Verification items for the finished model (mm, model axes). A direction names the side the tool comes from. Round coordinates to 2 decimals unless told otherwise and drop trailing zeros. Order: outer loops, then holes, each group sorted by start corner. A loop starts at its lowest first (then second) coordinate and runs counter-clockwise, first axis right, second up. Notation, with made-up numbers: M 85.25,-1.5 L 98.25,-1.5 A29 cw 98.25,27.5 Z; hole C 9,48 d2. An arc over 180 degrees is marked long. Use one line per item in the form item = value. Start each with the question number.
Item 1: Thickness scan on probe 1 along Z at (x, y) = (0, 506); probe 2 along Z at (x, y) = (68, 118.5); probe 3 along Y at (x, z) = (-36.5, -3.5). Record the ranges inside material, lowest first. Write a range as [from, to].
Item 2: Release check for a two-part mould opening along X. For faces 3 (the flat face through (-34, 0, -95)), 4 (the cylindrical face through (-89.42, 470.82, 37.07)), 5 (the cylindrical face through (138.304, -3.944, -43.554)), 6 (the flat face through (-1, 0, 1)) record: +X half, -X half, draft (parallel to the pull), parting line (faces both ways), or undercut.
Item 3: Cross-section at C-C on y = 176.5. Enter the section's corners in (x, z).
Item 4: Tool access check on faces 1 (the flat face through (52, 955, 82)), 2 (the cylindrical face through (-95.38, 470.82, -30.04)). Record the directions out of +Z, -Z, +X, -X, +Y, -Y that give a thin tool (end or side, any length) a straight path to the whole face; none if there is none.
Item 5: Cross-section at B-B on x = 0. Enter the section's corners in (y, z).
Item 6: Cross-section at A-A on z = 0. Enter the section's corners in (x, y), then the cut area to 3 significant figures.
Item 7: Go/stop test with flat-tipped pins: pin 1 Ø5 at (x, y) = (89.5, 847) entering from +Z; pin 2 Ø10 at (x, y) = (-10, 223.5) entering from +Z; pin 3 Ø3 at (y, z) = (638, 80.5) entering from +X. Record where each tip stops, or that it passes through.
Item 8: Cross-section at D-D on x = 110.5. Enter the section's corners in (y, z).
Autodesk Inventor part; units mm, degrees
ref_plane "YZ Plane" through (0, 0, 0) normal (1, 0, 0) x (0, 1, 0)
ref_plane "XZ Plane" through (0, 0, 0) normal (0, 1, 0) x (-1, 0, 0)
ref_plane "XY Plane" through (0, 0, 0) normal (0, 0, 1) x (1, 0, 0)
sketch "Boceto1" plane through (0, 0, 0) normal (0, 1, 0) x (-1, 0, 0)
  circle A0 centre (0, 0) radius 100
  circle A1 centre (0, 0) radius 96.8
  dimension "d0" = 200
  dimension "d1" = 193.6
extrude "Extrusión1" add sketch "Boceto1" along normal blind 955
sketch "Boceto2" plane through (0, 0, 0) normal (0, -1, 0) x (1, 0, 0)
  circle A0 centre (0, 0) radius 145
  dimension "d4" = 290
extrude "Extrusión2" add sketch "Boceto2" along normal blind 8
sketch "Boceto3" plane through (0, 955, 0) normal (0, 1, 0) x (1, 0, 0)
  point P0 (0, 0)
properties part number "Cuerpo"
Output values:
q1.probe_1 = [-100, -96.8], [96.8, 100]
q1.probe_2 = [-73.32, -68.89], [68.89, 73.32]
q1.probe_3 = [-8, 0]
q2.face_3 = draft
q2.face_4 = undercut
q2.face_5 = parting line
q2.face_6 = undercut
q3.outline = C 0,0 d200; hole C 0,0 d193.6
q4.face_1 = +Z, -Z, +X, -X, +Y
q4.face_2 = +Y
q5.outline = M -8,-145 L 0,-145 L 0,-100 L 955,-100 L 955,-96.8 L 0,-96.8 L 0,96.8 L 955,96.8 L 955,100 L 0,100 L 0,145 L -8,145 Z
q6.outline = M -145,-8 L 145,-8 L 145,0 L 100,0 L 100,955 L 96.8,955 L 96.8,0 L -96.8,0 L -96.8,955 L -100,955 L -100,0 L -145,0 Z
q6.area = 8,430 mm2
q7.pin_1 = 49.31
q7.pin_2 = 99.87
q7.pin_3 = 61.31
q8.outline = M -8,-93.89 L 0,-93.89 L 0,93.89 L -8,93.89 Z
